Geometry check sheet. Reference: the model listing, model coordinates, mm. Face numbers are marked on the shaded views. A direction names the side the tool comes from. Coordinates: 2 decimals unless noted, no trailing zeros. Write each loop counter-clockwise with the first axis right and the second up, starting at its lowest first coordinate (ties: lowest second). Pieces come first, ordered by that corner, then holes. Notation, with made-up numbers: M 74.5,-25 L 123.5,-25 A14 cw 123.5,-16 Z; hole C 43.5,58.5 d11. An arc over 180 degrees is marked long. Put each result on its own line as item: value. Start each with the question number.
1) Set-up check for the marked faces 4 and 5: record each of +Z, -Z, +X, -X, +Y, -Y from which the full face is reachable in a straight line by a thin tool's end or side.
2) Gauge pin test, flat ends, axial feed: pin 1 (3 mm diameter, centred on x = 67, y = 35, fed in from +Z); pin 2 (1 mm diameter, centred on x = 66.5, y = -29, fed in from +Z); pin 3 (8 mm diameter, centred on x = 29.5, z = 0.5, fed in from -Y); pin 4 (5 mm diameter, centred on y = 30, z = -6, fed in from -X). Record the tip position at first contact, or that the pin passes through.
3) Cross-section at B-B on x = 78. Record the cut outline in (y, z), plus the area to 3 significant figures.
4) Cross-section at A-A on z = 0. Record the cut outline in (x, y).
5) Mould release check, pull along Z, two halves, no side actions. Record for the marked faces 1, 2 and 3: released by +Z, released by -Z, zero draft, split by the parting line, or undercut.
6) Scan lines: line 1 along Z through (x, y) = (43.5, 2.5); line 2 along Y through (x, z) = (26, 4); line 3 along Y through (x, z) = (61.5, -2). Record each from-to range of solid material in increasing order.
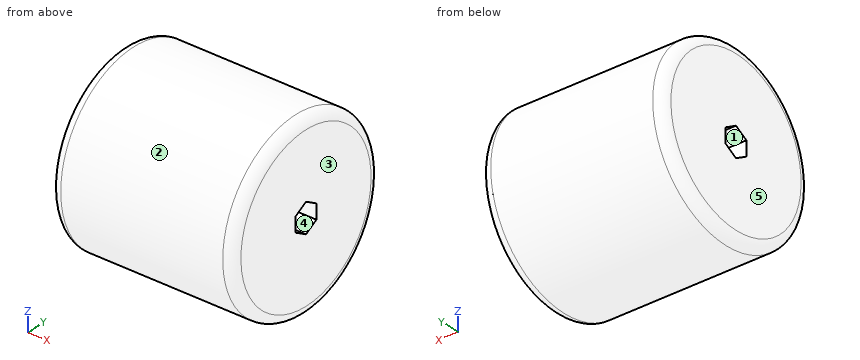
from build123d import *

# Parameters (mm, degrees)
CROQUIS1_R              = 44.77
SALIENTE_EXTRUIR1_DEPTH = 90.96
REDONDEO1_R             = 5


with BuildPart() as part:
    # Croquis1 → Saliente-Extruir1 (new body)
    with BuildSketch(Plane(origin=(0, 0, 0), x_dir=(0, 0, -1), z_dir=(1, 0, 0))):
        Circle(CROQUIS1_R)
        Polygon((7.332348419, 0), (3.666174209, 6.35), (-3.666174209, 6.35), (-7.332348419, 0), (-3.666174209, -6.35), (3.666174209, -6.35), align=None, mode=Mode.SUBTRACT)
    extrude(amount=SALIENTE_EXTRUIR1_DEPTH)

    # Redondeo1
    redondeo1_edges = [part.edges().sort_by_distance(p)[0] for p in [
        (0, 0, 44.77),
        (90.96, 0, 44.77),
    ]]
    fillet(redondeo1_edges, radius=REDONDEO1_R)


solid = part.part
Answer key:
1. face 4: +X, -X
1. face 5: +Z, -Z, -X, +Y, -Y
2. pin 1: stops at z = 29.7
2. pin 2: stops at z = 34.53
2. pin 3: stops at y = -44.77
2. pin 4: stops at x = 0
3. outline: C 0,0 d89.54; hole M -6.35,-3.67 L 0,-7.33 L 6.35,-3.67 L 6.35,3.67 L 0,7.33 L -6.35,3.67 Z
3. area: 6,160 mm²
4. outline: M 0,-39.77 A5 ccw 5,-44.77 L 85.96,-44.77 A5 ccw 90.96,-39.77 L 90.96,-6.35 L 0,-6.35 Z; M 0,6.35 L 90.96,6.35 L 90.96,39.77 A5 ccw 85.96,44.77 L 5,44.77 A5 ccw 0,39.77 Z
5. face 1: undercut
5. face 2: split by the parting line
5. face 3: zero draft
6. line 1: z = -44.7 to -5.89, 5.89 to 44.7
6. line 2: y = -44.59 to -5.77, 5.77 to 44.59
6. line 3: y = -44.73 to -6.35, 6.35 to 44.73
